from build123d import *

# Parameters (mm, degrees)
BOSS_EXTRUDE1_DEPTH = 50
SKETCH2_R           = 2.5
CUT_EXTRUDE2_DEPTH  = 50
SKETCH3_W           = 20
SKETCH3_H           = 20
BOSS_EXTRUDE2_DEPTH = 10
SKETCH4_R           = 8.769113897
BOSS_EXTRUDE3_DEPTH = 15
FILLET1_R           = 5
FILLET2_R           = 15
FILLET3_R           = 15
SKETCH7_R           = 3.769113897
BOSS_EXTRUDE4_DEPTH = 1
FILLET5_R           = 0.5


with BuildPart() as part:
    # Sketch1 → Boss-Extrude1 (new body)
    with BuildSketch(Plane(origin=(0, 0, 0), x_dir=(1, 0, 0), z_dir=(0, 1, 0))):
        Polygon((0, 0), (50, 0), (50, 50), (40, 50), (40, 10), (0, 10), align=None)
    extrude(amount=BOSS_EXTRUDE1_DEPTH)

    # Sketch2 → Cut-Extrude2 (cut)
    with BuildSketch(Plane.ZY.offset(-40)):
        with Locations((-40, 10)):
            Circle(SKETCH2_R)
        with Locations((-40, 40)):
            Circle(SKETCH2_R)
    extrude(amount=-CUT_EXTRUDE2_DEPTH, mode=Mode.SUBTRACT)

    # Sketch3 → Boss-Extrude2 (add)
    with BuildSketch(Plane.XY):
        with Locations((25, 25)):
            Rectangle(SKETCH3_W, SKETCH3_H)
    extrude(amount=BOSS_EXTRUDE2_DEPTH)

    # Sketch4 → Boss-Extrude3 (add)
    with BuildSketch(Plane.XY.offset(10)):
        with Locations((25, 25)):
            Circle(SKETCH4_R)
    extrude(amount=BOSS_EXTRUDE3_DEPTH)

    # Fillet1
    fillet1_edges = [part.edges().sort_by_distance(p)[0] for p in [
        (16.230886103, 25, 25),
    ]]
    fillet(fillet1_edges, radius=FILLET1_R)

    # Fillet2
    fillet2_edges = [part.edges().sort_by_distance(p)[0] for p in [
        (40, 25, -10),
    ]]
    fillet(fillet2_edges, radius=FILLET2_R)

    # Fillet3
    fillet3_edges = [part.edges().sort_by_distance(p)[0] for p in [
        (50, 25, 0),
    ]]
    fillet(fillet3_edges, radius=FILLET3_R - 0.0001)  # a hair under: the kernel refuses the full size

    # Sketch7 → Boss-Extrude4 (add)
    with BuildSketch(Plane.XY.offset(25)):
        with Locations((25, 25)):
            Circle(SKETCH7_R)
    extrude(amount=BOSS_EXTRUDE4_DEPTH)

    # Fillet5
    fillet5_edges = [part.edges().sort_by_distance(p)[0] for p in [
        (21.230886103, 25, 26),
    ]]
    fillet(fillet5_edges, radius=FILLET5_R)


solid = part.part
Could you check a few things on this model? Use its own coordinates, in mm. A direction names the side the tool comes from. Give positions to 0.01 mm unless a question says otherwise; leave off trailing zeros. Order: outer loops, then holes, each group sorted by start corner. A loop starts at its lowest first (then second) coordinate and runs counter-clockwise, first axis right, second up. Notation, with made-up numbers: (-28.5, -33.5) - (-1.5, -33.5) arc R18 ccw to (-1.5, -21.5) - close; hole circle Ø11 at (-17.75, 86.5). An arc over 180 degrees is marked (long way). Return JSON: item names as keys, results as strings. Group by question number.
Q1. Suppose I cut it at B-B, the plane z = -40. Please give me the cut outline in (x, y), and give its area (3 significant figures).
Q2. Thinking about a two-plate mould opening in Z: for faces 1 (the face through (35.49, 25.35, -14.28)), 2 (the face through (40, 25, -38)), 3 (the face through (44.93, 9.04, -37.69)), which applies, pulls with the +Z half, pulls with the -Z half, needs draft (parallel to the pull), parting line crosses it, or undercut?
Q3. Suppose I cut it at A-A, the plane y = 40. Please give me the cut outline in (x, z), and give its area (3 significant figures).
Q4. Please list where these lines run through material, in increasing order: line 1 along Y through (x, z) = (44.5, -40); line 2 along Z through (x, y) = (14.5, 18.5); line 3 along Y through (x, z) = (19, 2.5). Write a range as [from, to].
Q5. Suppose I cut it at C-C, the plane z = -13. Please give me the cut outline in (x, y), and give its area (3 significant figures).
Q6. Which directions (+Z, -Z, +X, -X, +Y, -Y) give clear straight access to the entire face, cutting with the end or side of a thin tool? Please do faces 4 (the face through (22.222, 27.547, 25.246)), 5 (the face through (15, 25, 5)), 6 (the face through (13, 25, -10)), 7 (the face through (35, 25, 5)), 8 (the face through (25, 15, 5)).
Q7. Will these pins go through, and if not, where does the flat tip stop? pin 1 Ø11 at (y, z) = (21, 6) entering from -X; pin 2 Ø8 at (x, y) = (17.5, 30) entering from -Z; pin 3 Ø3 at (y, z) = (26.5, 6) entering from +X.
Resolved:
{
 "1": {"outline": "(40, 0) - (50, 0) - (50, 7.5) - (40, 7.5) - close; (40, 12.5) - (50, 12.5) - (50, 37.5) - (40, 37.5) - close; (40, 42.5) - (50, 42.5) - (50, 50) - (40, 50) - close", "area": "400 mm2"},
 "2": {"face 1": "pulls with the -Z half", "face 2": "needs draft", "face 3": "undercut"},
 "3": {"outline": "(0, -10) - (25, -10) arc R15 cw to (40, -25) - (40, -37.5) - (50, -37.5) - (50, -15) arc R15 ccw to (35, 0) - (0, 0) - close; (40, -50) - (50, -50) - (50, -42.5) - (40, -42.5) - close", "area": "850 mm2"},
 "4": {"line 1": "y = [0, 7.5], [12.5, 37.5], [42.5, 50]", "line 2": "z = [-10, 0]", "line 3": "y = [15, 35]"},
 "5": {"outline": "(34, 0) - (49.87, 0) - (49.87, 50) - (34, 50) - close", "area": "793 mm2"},
 "6": {"face 4": "+Z", "face 5": "+Z, -X, +Y, -Y", "face 6": "-Z, -X, +Y, -Y", "face 7": "+Z, +X, +Y, -Y", "face 8": "+Z, +X, -X, -Y"},
 "7": {"pin 1": "stops at x = 15", "pin 2": "stops at z = -10", "pin 3": "stops at x = 35"}
}
